CAD build for the part. Positions are in the model's coordinates, mm. A direction names the side the tool comes from. Give positions to 0.01 mm unless a question says otherwise; leave off trailing zeros. Write each loop counter-clockwise with the first axis right and the second up, starting at its lowest first coordinate (ties: lowest second). Pieces come first, ordered by that corner, then holes. Notation, with made-up numbers: (-29.5, 72) -> (-16.5, 72) arc R21 cw to (-16.5, 104) -> close; hole circle Ø9 at (24.25, -3). An arc over 180 degrees is marked (long way). Answer as a JSON object with one key per item and string values.
```python
from build123d import *

# Parameters (mm, degrees)
F1_DEPTH = 6.35
F2_W     = 15.6363076478
F2_H     = 33.7427960873
F3_DEPTH = 101.6


with BuildPart() as f1:
    # F0 (on Top) → F1 (new body, symmetric)
    with BuildSketch(Plane.XY):
        Polygon((38.1, 50.8), (0, 50.8), (-38.1, 50.8), (-38.1, 0), (-38.1, -50.8), (0, -50.8), (38.1, -50.8), (38.1, 0), align=None)
    extrude(amount=F1_DEPTH, both=True)

    # F2 (on face) → F3 (join)
    with BuildSketch(Plane.XZ.offset(50.8)):
        with Locations((-30.2818461761, 23.2213980436)):
            Rectangle(F2_W, F2_H)
    extrude(amount=-F3_DEPTH)

    # F4: F1 across plane


with BuildPart() as f1_1:
    add(f1.part)
    add(f1.part.mirror(Plane.YZ))


solid = f1_1.part
```
1) Slice it at C-C (x = -4.5). List the corners of the cut face in (y, z).
Model answer:
{"outline": "(-50.8, -6.35) -> (50.8, -6.35) -> (50.8, 6.35) -> (-50.8, 6.35) -> close"}
2) Wall check: probe 1 along X at (y, z) = (21.5, 8); probe 2 along Z at (x, y) = (-11, 4.5). Give the ranges that are in metal, low to high.
Model answer:
{"probe 1": "x = -38.1 to -22.46, 22.46 to 38.1", "probe 2": "z = -6.35 to 6.35"}
3) Pin check, flat tip, straight feed: pin 1 (10 mm diameter, centred on x = 14.5, z = 35, fed in from -Y). Stop position of the tip, or through.
Model answer:
{"pin 1": "passes through"}
4) Mould opens along X. For faces 3 (the flat face through (-38.1, -1, 17)), 4 (the flat face through (-1, 1, -6.35)), 5 (the flat face through (0, 1, 6.35)) say: released by +X, released by -X, zero draft, split by the parting line, or undercut.
Model answer:
{"face 3": "released by -X", "face 4": "zero draft", "face 5": "undercut"}
5) 3-axis set-ups, long thin cutter, end or side, ignore diameter. For faces 1 (the flat face through (22.464, -1, 23)), 2 (the flat face through (1, 50.8, 2)): which of +Z, -Z, +X, -X, +Y, -Y reach the whole face in a straight line?
Model answer:
{"face 1": "+Z, +Y, -Y", "face 2": "+Z, -Z, +X, -X, +Y"}
6) Slice it at B-B (y = -3). List the corners of the cut face in (x, z).
Model answer:
{"outline": "(-38.1, -6.35) -> (38.1, -6.35) -> (38.1, 40.09) -> (22.46, 40.09) -> (22.46, 6.35) -> (-22.46, 6.35) -> (-22.46, 40.09) -> (-38.1, 40.09) -> close"}
7) Slice it at A-A (z = 32). List the corners of the cut face in (x, y).
Model answer:
{"outline": "(-38.1, -50.8) -> (-22.46, -50.8) -> (-22.46, 50.8) -> (-38.1, 50.8) -> close; (22.46, -50.8) -> (38.1, -50.8) -> (38.1, 50.8) -> (22.46, 50.8) -> close"}
